Answer from the drawing. Dimensions are ordinates in mm from the lowest x, y and z of the part. Round coordinates to 2 decimals unless told otherwise and drop trailing zeros. Order: outer loops, then holes, each group sorted by start corner. A loop starts at its lowest first (then second) coordinate and runs counter-clockwise, first axis right, second up. Notation, with made-up numbers: (-34, -24) -> (-20, -24) arc R32 cw to (-20, 15) -> close; hole circle Ø1 at (-4, -16). An arc over 180 degrees is marked (long way). Use a Markdown table: item, result. Add a question column.
Item 1: A cutting plane is placed at C-C, the plane x = 55. Determine the outline of the cut face in (y, z), plus the area to 3 significant figures.
Item 2: A cutting plane is placed at B-B, the plane y = 65. Determine the outline of the cut face in (x, z).
Item 3: A cutting plane is placed at A-A, the plane z = 1.6. Determine the outline of the cut face in (x, y), plus the area to 3 significant figures.
Item 4: Find the intervals of material crossed by L1, parallel to X at y = 61.5, z = 0.75; L2, parallel to Y at x = 10, z = 0.25; L3, parallel to Y at x = 36.5, z = 1.35, in increasing order. Write a range as [from, to].
Item 5: A flat-ended cylindrical pin translates along its axis: P1, Ø1, axis at x = 48.5, z = 1.5, coming from the -Y side. Find the tip coordinate at first contact, or state that the pin passes through.
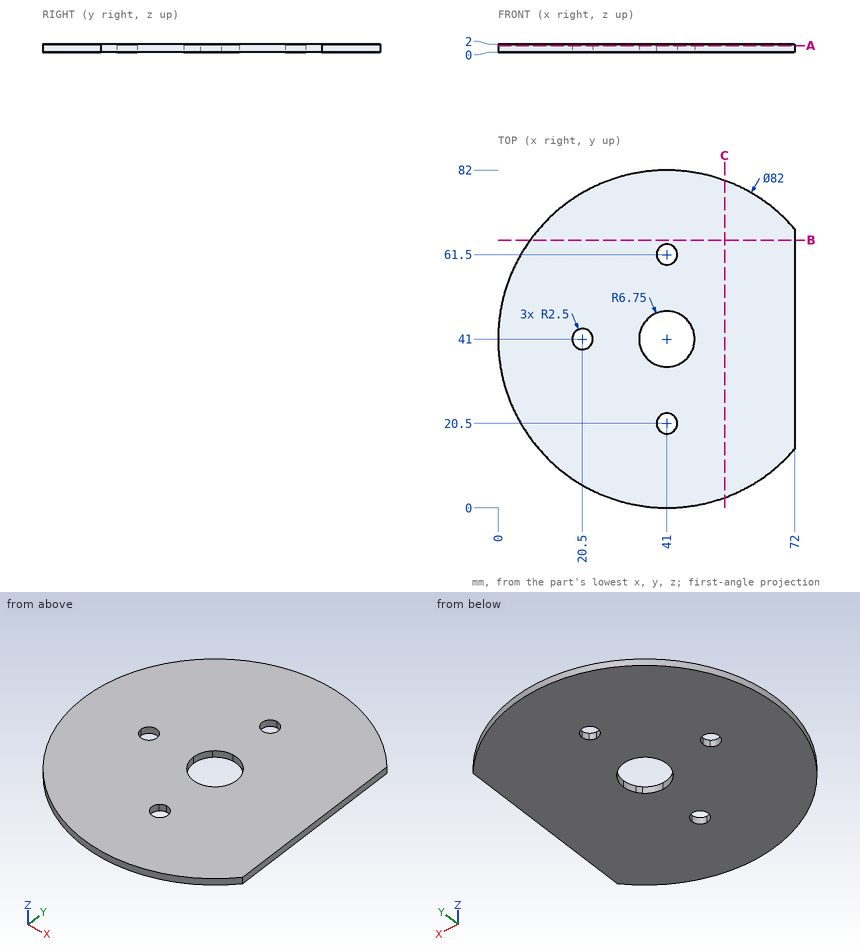
Reported:
| question | item | result |
|---|---|---|
| 1 | outline | (2.46, 0) -> (79.54, 0) -> (79.54, 2) -> (2.46, 2) -> close |
| 1 | area | 154 mm² |
| 2 | outline | (7.76, 0) -> (72, 0) -> (72, 2) -> (7.76, 2) -> close |
| 3 | outline | (72, 14.17) -> (72, 67.83) arc R41 ccw (long way) to start; hole circle Ø5 at (20.5, 41); hole circle Ø13.5 at (41, 41); hole circle Ø5 at (41, 20.5); hole circle Ø5 at (41, 61.5) |
| 3 | area | 4,710 mm² |
| 4 | L1 | [5.49, 38.5], [43.5, 72] |
| 4 | L2 | [14.17, 67.83] |
| 4 | L3 | [0.25, 35.97], [46.03, 81.75] |
| 5 | P1 | y = 0.6 |
